For this review, take the finished solid that the model builds, in its own axes (mm). Face numbers are marked on the shaded views. A direction names the side the tool comes from. Coordinates: 2 decimals unless noted, no trailing zeros. Write each loop counter-clockwise with the first axis right and the second up, starting at its lowest first coordinate (ties: lowest second). Pieces come first, ordered by that corner, then holes.
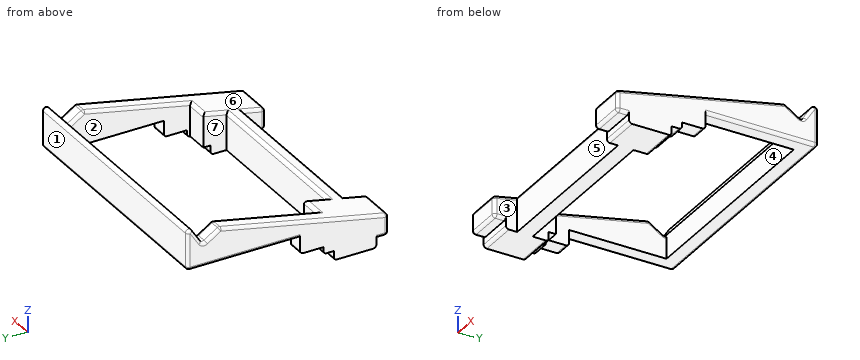
```python
from build123d import *

# Parameters (mm, degrees)
PAD_DEPTH         = 160
FILLET_R          = 2
SKETCH001_W       = 15
SKETCH001_H       = 111
POCKET_DEPTH      = 25.547835
POCKET_DEPTH_BACK = -21.001
FILLET001_R       = 2


with BuildPart() as part:
    # Sketch → Pad (new body)
    with BuildSketch(Plane.YZ):
        with BuildLine():
            Line((0, 0), (0, 13.384276))
            Line((0, 13.384276), (108.603536, 36.46867))
            Line((108.603536, 36.46867), (117.942463, 30.4039))
            ThreePointArc((117.942463, 30.4039), (119.447565, 30.124946), (120.709082, 30.991963))
            Line((120.709082, 30.991963), (126.322659, 39.636113))
            ThreePointArc((130, 38.546835), (128.568031, 40.464474), (126.322659, 39.636113))
            Line((130, 38.546835), (130, 15))
            Line((130, 15), (57, 15))
            Line((57, 15), (57, 4.5))
            Line((57, 4.5), (42, 4.5))
            Line((42, 4.5), (42, 0))
            Line((42, 0), (35.25, 0))
            Line((35.25, 0), (35.25, -6))
            Line((35.25, -6), (7.75, -6))
            Line((7.75, -6), (7.75, 0))
            Line((7.75, 0), (0, 0))
        make_face()
    extrude(amount=PAD_DEPTH)

    # Fillet
    fillet_edges = [part.edges().sort_by_distance(p)[0] for p in [
        (80, 42, 0),
        (80, 35.25, -6),
        (80, 0, 13.384276),
        (80, 108.603536, 36.46867),
        (80, 130, 38.546835),
        (80, 130, 15),
        (80, 0, 0),
        (80, 57, 4.5),
        (80, 7.75, -6),
    ]]
    fillet(fillet_edges, radius=FILLET_R)

    # Sketch001 (on Face2 of Pad) → Pocket (cut, two sides)
    with BuildSketch(Plane.YX.offset(-15)) as pocket_sk:
        Polygon((25, 135.5), (25, 24.5), (40, 24.5), (40, 10), (120, 10), (120, 150), (40, 150), (40, 135.5), align=None)
        with Locations((7.5, 80)):
            Rectangle(SKETCH001_W, SKETCH001_H)
    extrude(amount=-POCKET_DEPTH, mode=Mode.SUBTRACT)
    extrude(pocket_sk.sketch, amount=-POCKET_DEPTH_BACK, mode=Mode.SUBTRACT)

    # Fillet001
    fillet001_edges = [part.edges().sort_by_distance(p)[0] for p in [
        (0, 54.688694, 25.008717),
        (160, 54.688694, 25.008717),
        (150, 73.896606, 29.091484),
        (10, 73.896606, 29.091484),
        (80, 25, 18.69819),
        (80, 15, 16.572624),
        (24.5, 0, 6.882354),
        (135.5, 0, 6.882354),
        (24.5, 32.5, 20.292364),
        (135.5, 32.5, 20.292364),
        (142.75, 40, 21.886538),
        (17.25, 40, 21.886538),
    ]]
    fillet(fillet001_edges, radius=FILLET001_R)


solid = part.part
```
1) Consider section A-A (x = 97). Give the boundary of the cut face in (y, z), then the cut area to 3 significant figures.
2) The part is to be moulded in two halves that separate along Y. For the marked faces 1, 2, 3 and 4, say which applies: pulls with the +Y half, pulls with the -Y half, needs draft (parallel to the pull), parting line crosses it, or undercut.
3) Clearance check with flat-ended pins moving along their axes: P1, Ø3, axis at x = 5, z = 12.5, coming from the +Y side; P2, Ø5, axis at x = 4.5, y = 47.5, coming from the -Z side; P3, Ø1.5, axis at x = 23, z = 0.5, coming from the +Y side; P4, Ø8, axis at y = 60.5, z = 31.5, coming from the +X side. State where each tip first meets the part, or that it passes through.
4) For L1, parallel to X at y = 94.5, z = 24; L2, parallel to Y at x = 123, z = 6; L3, parallel to X at y = 30, z = 3.5, list the stretches that pass through material, from the lowest coordinate up.
5) Tool access review of the marked faces 5, 6 and 7: name each direction out of +Z, -Z, +X, -X, +Y, -Y from which nothing blocks a thin tool from reaching the whole face with its end or side.
Results:
1. outline: (15, -6) - (25, -6) - (25, 16.23) arc R2 ccw to (22.58, 18.18) - (16.58, 16.91) arc R2 ccw to (15, 14.95) - close; (120, 15) - (128, 15) arc R2 ccw to (130, 17) - (130, 38.55) arc R2 ccw to (126.32, 39.64) - (120.71, 30.99) arc R2 cw to (120, 30.33) - close
1. area: 451 mm2
2. face 1: pulls with the +Y half
2. face 2: undercut
2. face 3: needs draft
2. face 4: undercut
3. P1: stops at y = 57
3. P2: stops at z = 4.5
3. P3: stops at y = 40
3. P4: passes through
4. L1: x = 0 to 10, 150 to 160
4. L2: y = 15 to 25
4. L3: x = 0 to 24.5, 135.5 to 160
5. face 5: +Z, -Z, -Y
5. face 6: +Z, +X, -X, -Y
5. face 7: +Z, -Z
